```python
from build123d import *

# Parameters (mm, degrees)
SKETCH1_W               = 635
SKETCH1_H               = 101.6
BOSS_EXTRUDE1_DEPTH     = 28.448
CUT_EXTRUDE1_START      = -29.448
SKETCH1_3_R             = 12.7
CUT_EXTRUDE1_DEPTH      = 30.448
LPATTERN1_COUNT         = 16
LPATTERN1_PITCH         = 36.83
SKETCH3_R               = 12.7
CUT_EXTRUDE2_DEPTH      = 1
CUT_EXTRUDE2_DEPTH_BACK = 29.448


with BuildPart() as part:
    # Sketch1 → Boss-Extrude1 (new body)
    with BuildSketch(Plane.XY):
        with Locations((-280.035, 2.75844)):
            Rectangle(SKETCH1_W, SKETCH1_H)
    extrude(amount=-BOSS_EXTRUDE1_DEPTH)

    # Sketch1<3> → Cut-Extrude1 (cut)
    with BuildSketch(Plane.XY.offset(CUT_EXTRUDE1_START)):
        Circle(SKETCH1_3_R)
        with Locations((18.415, 31.89478)):
            Circle(SKETCH1_3_R)
        with Locations((18.415, -31.89478)):
            Circle(SKETCH1_3_R)
    cut_extrude1 = extrude(amount=CUT_EXTRUDE1_DEPTH, mode=Mode.SUBTRACT)

    # LPattern1: Cut-Extrude1 ×16
    with Locations(*[(-i * LPATTERN1_PITCH, 0, 0) for i in range(1, LPATTERN1_COUNT)]):
        add(cut_extrude1, mode=Mode.SUBTRACT)

    # Sketch3 → Cut-Extrude2 (cut, two sides)
    with BuildSketch(Plane.XY) as cut_extrude2_sk:
        with Locations((-570.865, 31.89478)):
            Circle(SKETCH3_R)
        with Locations((-570.865, -31.89478)):
            Circle(SKETCH3_R)
    extrude(amount=CUT_EXTRUDE2_DEPTH, mode=Mode.SUBTRACT)
    extrude(cut_extrude2_sk.sketch, amount=-CUT_EXTRUDE2_DEPTH_BACK, mode=Mode.SUBTRACT)


solid = part.part
```
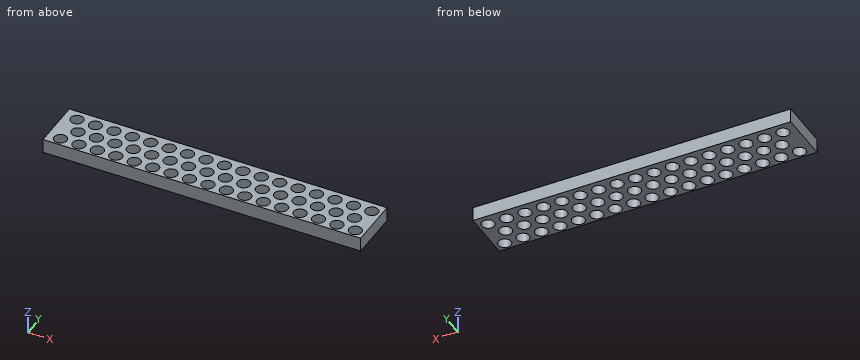
Geometry: final body of the model. Coordinates: model frame, mm. Coordinates: 2 decimals unless noted, no trailing zeros. Order: outer loops, then holes, each group sorted by start corner. A loop starts at its lowest first (then second) coordinate and runs counter-clockwise, first axis right, second up. Notation, with made-up numbers: M -7,-39.5 L 45,-39.5 A18 cw 45,-4.5 Z; hole C 3,19 d10. An arc over 180 degrees is marked long. Answer in a Markdown table with one row per item. Add a question column.
Q1. Section query A-A on x = -147.32. Return the cut outline in (y, z), and give its area (3 significant figures).
Q2. Line query: L1, parallel to Y at x = -388.5, z = -12; L2, parallel to Y at x = -93, z = -4.5; L3, parallel to Y at x = -44, z = -17.5. Output: solid intervals per line, ascending.
Q3. Section query B-B on y = 7.5. Count the separate pieces of the cut face and the enclosed holes in it, and give its area (3 significant figures).
Completed:
| question | item | result |
|---|---|---|
| 1 | outline | M -48.04,-28.45 L -12.7,-28.45 L -12.7,0 L -48.04,0 Z; M 12.7,-28.45 L 53.56,-28.45 L 53.56,0 L 12.7,0 Z |
| 1 | area | 2,170 mm2 |
| 2 | L1 | y = -48.04 to -44.47, -19.32 to 19.32, 44.47 to 53.56 |
| 2 | L2 | y = -48.04 to -44.56, -19.23 to 19.23, 44.56 to 53.56 |
| 2 | L3 | y = -48.04 to -37.8, -25.99 to -10.48, 10.48 to 25.99, 37.8 to 53.56 |
| 3 | separate pieces | 17 |
| 3 | enclosed holes | 0 |
| 3 | area | 8,730 mm2 |
